```python
from build123d import *

# Parameters (mm, degrees)
SKETCH1_R           = 2.5
BOSS_EXTRUDE1_DEPTH = 10
SKETCH2_R           = 1.75
BOSS_EXTRUDE2_DEPTH = 24
CHAMFER1_SIZE       = 1.5
CHAMFER1_SIZE2      = 8.506922729


with BuildPart() as part:
    # Sketch1 → Boss-Extrude1 (new body)
    with BuildSketch(Plane(origin=(0, 0, 0), x_dir=(0, 0, -1), z_dir=(1, 0, 0))):
        Circle(SKETCH1_R)
    extrude(amount=BOSS_EXTRUDE1_DEPTH)

    # Sketch2 → Boss-Extrude2 (add)
    with BuildSketch(Plane(origin=(10, 0, 0), x_dir=(0, 0, -1), z_dir=(1, 0, 0))):
        Circle(SKETCH2_R)
    extrude(amount=BOSS_EXTRUDE2_DEPTH)

    # Chamfer1
    chamfer1_edges = [part.edges().sort_by_distance(p)[0] for p in [
        (34, 0, 1.75),
    ]]
    chamfer1_side = [part.faces().sort_by_distance(p)[0] for p in [
        (34, 0, 0),
    ]]
    chamfer(chamfer1_edges, length=CHAMFER1_SIZE, length2=CHAMFER1_SIZE2, reference=chamfer1_side[0])


solid = part.part
```
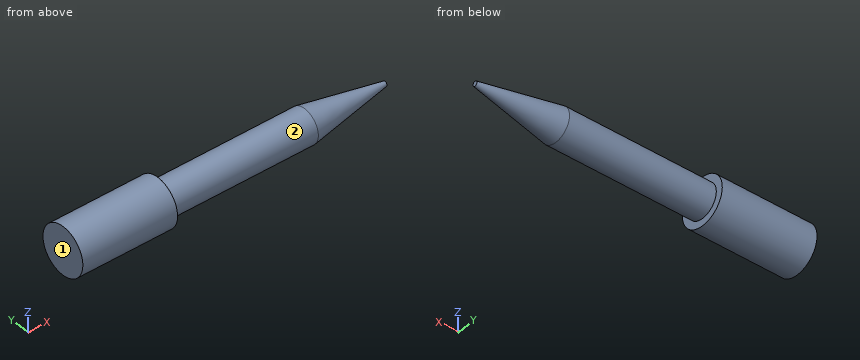
Check sheet for the modelled part. Datum: model origin and axes. Units: mm. Face numbers are marked on the shaded views. A direction names the side the tool comes from. Round coordinates to 2 decimals unless told otherwise and drop trailing zeros. Loops run counter-clockwise (first coordinate to the right, second up) from the corner with the lowest first, then second, coordinate; pieces in that order, holes last. Notation, with made-up numbers: (77, 0) - (83, 0) arc R16 ccw to (83, 4) - close; hole circle Ø1 at (-15.5, 55.5). An arc over 180 degrees is marked (long way). Write item = value, one per line. Start each with the question number.
Q1. Access from +Z, -Z, +X, -X, +Y, -Y to the whole of each face (thin tool, end or side, straight path). Record for the marked faces 1 and 2.
Q2. Section check A-A (x = 18). Record the boundary of the cut face in (y, z).
Q3. Depth check by flat-ended pin: P1, Ø3, axis at y = 1.5, z = -0.5, coming from the +X side; P2, Ø1.5, axis at x = 21, y = 0, coming from the +Z side. Enter the tip coordinate at first touch or a pass-through.
Q4. Thickness scan on L1, parallel to X at y = 2, z = 0.7; L2, parallel to Z at x = 24.5, y = 0.4; L3, parallel to Y at x = 23.5, z = 0.75. Record the ranges inside material, lowest first.
Q5. Section check B-B (x = 8). Record the boundary of the cut face in (y, z), plus the area to 3 significant figures.
Derived:
q1.face_1 = +Z, -Z, -X, +Y, -Y
q1.face_2 = +X
q2.outline = circle Ø3.5 at (0, 0)
q3.P1 = 34
q3.P2 = 1.75
q4.L1 = 0 to 10
q4.L2 = -1.7 to 1.7
q4.L3 = -1.58 to 1.58
q5.outline = circle Ø5 at (0, 0)
q5.area = 19.6 mm^2
